Input: part model. Units: mm. Frame: model coordinates. A direction names the side the tool comes from. Give positions to 0.01 mm unless a question says otherwise; leave off trailing zeros. Loops run counter-clockwise (first coordinate to the right, second up) from the corner with the lowest first, then second, coordinate; pieces in that order, holes last. Notation, with made-up numbers: M 39,-7.75 L 59,-7.75 A20 cw 59,0.25 Z; hole C 44,63.25 d6. An arc over 180 degrees is marked long. Use CSV: the item, a comma, the result in double quotes. Start each with the question number.
Autodesk Inventor part; units mm, degrees
ref_plane "YZ Plane" through (0, 0, 0) normal (1, 0, 0) x (0, 1, 0)
ref_plane "XZ Plane" through (0, 0, 0) normal (0, 1, 0) x (-1, 0, 0)
ref_plane "XY Plane" through (0, 0, 0) normal (0, 0, 1) x (1, 0, 0)
sketch "Boceto1" plane through (0, 0, 0) normal (0, 0, 1) x (1, 0, 0)
  arc A0 (168.6959, -21.0168) -> (169.5218, -12.7418) centre (0, 0) ccw
  arc A1 (169.5218, -12.7418) -> (124.9741, 2.5458) centre (132.4533, -48.2091) ccw
  arc A2 (122.0053, -27.1977) -> (168.6959, -21.0168) centre (139.3691, 21.0776) ccw
  arc A3 (162.6596, 49.415) -> (160.0484, 57.3105) centre (0, 0) ccw
  arc A4 (160.0484, 57.3105) -> (113.134, 53.1573) centre (140.6105, 9.8324) ccw
  arc A5 (122.5196, 24.7777) -> (162.6596, 49.415) centre (118.7469, 75.9418) ccw
  arc A6 (128.4981, 111.3025) -> (122.9012, 117.4533) centre (0, 0) ccw
  arc A7 (122.9012, 117.4533) -> (81.7321, 94.5773) centre (124.4549, 66.1738) ccw
  arc A8 (101.8493, 72.4688) -> (128.4981, 111.3025) centre (77.5924, 117.6751) ccw
  arc A9 (72.1181, 153.9447) -> (64.5033, 157.2874) centre (0, 0) ccw
  arc A10 (64.5033, 157.2874) -> (36.1979, 119.6441) centre (86.7799, 111.0732) ccw
  arc A11 (63.5682, 107.6294) -> (72.1181, 153.9447) centre (23.0214, 139.0612) ccw
  arc A12 (3.2682, 169.9686) -> (-5.0479, 169.925) centre (0, 0) ccw
  arc A13 (-5.0479, 169.925) -> (-15.5952, 124.0233) centre (34.0998, 136.767) ccw
  arc A14 (14.2956, 124.1798) -> (3.2682, 169.9686) centre (-35.5302, 136.4024) ccw
  arc A15 (-66.1468, 156.6033) -> (-73.7262, 153.1811) centre (0, 0) ccw
  arc A16 (-73.7262, 153.1811) -> (-64.6918, 106.9578) centre (-24.4764, 138.8125) ccw
  arc A17 (-37.4488, 119.2585) -> (-66.1468, 156.6033) centre (-87.9383, 110.1584) ccw
  arc A18 (-124.1244, 116.1599) -> (-129.6566, 109.9508) centre (0, 0) ccw
  arc A19 (-129.6566, 109.9508) -> (-102.6026, 71.3983) centre (-78.8204, 116.8561) ccw
  arc A20 (-82.718, 93.7163) -> (-124.1244, 116.1599) centre (-125.141, 64.867) ccw
  arc A21 (-160.6398, 55.6314) -> (-163.1682, 47.7089) centre (0, 0) ccw
  arc A22 (-163.1682, 47.7089) -> (-122.7724, 23.4934) centre (-119.5357, 74.6942) ccw
  arc A23 (-113.6845, 51.9696) -> (-160.6398, 55.6314) centre (-140.7058, 8.3595) ccw
  arc A24 (-169.3791, -14.5163) -> (-168.4665, -22.7822) centre (0, 0) ccw
  arc A25 (-168.4665, -22.7822) -> (-121.7138, -28.4738) centre (-139.5821, 19.617) ccw
  arc A26 (-124.9939, 1.237) -> (-169.3791, -14.5163) centre (-131.9412, -49.5935) ccw
  arc A27 (-148.8312, -82.154) -> (-144.6355, -89.3341) centre (0, 0) ccw
  arc A28 (-144.6355, -89.3341) -> (-99.6097, -75.5175) centre (-135.4936, -38.8522) ccw
  arc A29 (-114.6907, -49.7095) -> (-148.8312, -82.154) centre (-100.3628, -98.9712) ccw
  arc A30 (-102.549, -135.5865) -> (-95.7956, -140.4393) centre (0, 0) ccw
  arc A31 (-95.7956, -140.4393) -> (-60.2823, -109.5036) centre (-107.9769, -90.6034) ccw
  arc A32 (-84.5565, -92.0608) -> (-102.549, -135.5865) centre (-51.4308, -131.2359) ccw
  arc A33 (-38.5352, -165.5749) -> (-30.3919, -167.2613) centre (0, 0) ccw
  arc A34 (-30.3919, -167.2613) -> (-10.5315, -124.5556) centre (-61.7901, -126.6885) ccw
  arc A35 (-39.8017, -118.494) -> (-38.5352, -165.5749) centre (6.3941, -140.8088) ccw
  arc A36 (32.1417, -166.9339) -> (40.267, -165.1623) centre (0, 0) ccw
  arc A37 (40.267, -165.1623) -> (41.0403, -118.0707) centre (-4.9192, -140.868) ccw
  arc A38 (11.8352, -124.4385) -> (32.1417, -166.9339) centre (63.1134, -126.0345) ccw
  arc A39 (97.261, -139.4285) -> (103.9632, -134.5052) centre (0, 0) ccw
  arc A40 (103.9632, -134.5052) -> (85.5159, -91.1703) centre (52.8023, -130.6902) ccw
  arc A41 (61.4257, -108.8664) -> (97.261, -139.4285) centre (108.9198, -89.4677) ccw
  arc A42 (145.563, -87.8146) -> (149.6833, -80.5909) centre (0, 0) ccw
  arc A43 (149.6833, -80.5909) -> (115.205, -48.5058) centre (101.3937, -97.9148) ccw
  arc A44 (100.3951, -74.4703) -> (145.563, -87.8146) centre (135.893, -37.4312) ccw
  arc A45 (113.134, 53.1573) -> (101.8493, 72.4688) centre (0, 0) ccw
  arc A46 (124.9741, 2.5458) -> (122.5196, 24.7777) centre (0, 0) ccw
  arc A47 (115.205, -48.5058) -> (122.0053, -27.1977) centre (0, 0) ccw
  arc A48 (85.5159, -91.1703) -> (100.3951, -74.4703) centre (0, 0) ccw
  arc A49 (41.0403, -118.0707) -> (61.4257, -108.8664) centre (0, 0) ccw
  arc A50 (-10.5315, -124.5556) -> (11.8352, -124.4385) centre (0, 0) ccw
  arc A51 (-60.2823, -109.5036) -> (-39.8017, -118.494) centre (0, 0) ccw
  arc A52 (-99.6097, -75.5175) -> (-84.5565, -92.0608) centre (0, 0) ccw
  arc A53 (-121.7138, -28.4738) -> (-114.6907, -49.7095) centre (0, 0) ccw
  arc A54 (-122.7724, 23.4934) -> (-124.9939, 1.237) centre (0, 0) ccw
  arc A55 (-102.6026, 71.3983) -> (-113.6845, 51.9696) centre (0, 0) ccw
  arc A56 (-64.6918, 106.9578) -> (-82.718, 93.7163) centre (0, 0) ccw
  arc A57 (-15.5952, 124.0233) -> (-37.4488, 119.2585) centre (0, 0) ccw
  arc A58 (81.7321, 94.5773) -> (63.5682, 107.6294) centre (0, 0) ccw
  arc A59 (36.1979, 119.6441) -> (14.2956, 124.1798) centre (0, 0) ccw
  dimension "d8" = 360
extrude "Extrusión1" add sketch "Boceto1" along normal blind 30
properties part number "15P_Recto"
Item 1: Section B-B (y = -65). Output: boundary loops of the cut face in (x, z), then the cut area to 3 significant figures.
Item 2: Material intervals for line 1 (Y direction, x = -122.5, z = 3.75); line 2 (Y direction, x = -135, z = 23); line 3 (X direction, y = 135, z = 15.25), sorted ascending.
Item 3: Set-up query: faces 5 (the cylindrical face through (-120.62, 87.11, 14.79)), 6 (the cylindrical face through (72.82, 101.6, 14.79)). Return all of +Z, -Z, +X, -X, +Y, -Y with unobstructed straight access to the full face (end or side cutting, diameter ignored); none if empty.
Item 4: First-contact query: pin 1 Ø2 at (y, z) = (21.5, 5.5) entering from -X; pin 2 Ø8 at (y, z) = (-87, 8) entering from -X; pin 3 Ø3 at (x, z) = (13, 26) entering from +Y. Flat tips, straight axial feed; report the tip coordinate or a pass-through.
Item 5: Mould query, pull axis X, two halves, no side actions, for faces 1 (the cylindrical face through (-47.47, 141.69, 14.79)), 2 (the cylindrical face through (169.165, -16.826, 14.79)), 3 (the cylindrical face through (16.97, -148.46, 14.79)), 4 (the flat face through (-2, 4, 0)). Classes: +X half, -X half, draft (parallel to the pull), parting line (faces both ways), or undercut.
Item 6: Section A-A (y = 67.5). Output: boundary loops of the cut face in (x, z), then the cut area to 3 significant figures.
Recorded:
1,outline,"M -138.81,0 L 140.75,0 L 140.75,30 L -138.81,30 Z"
1,area,"8,390 mm²"
2,line 1,"-88.48 to -52.69, -28.76 to 56.32, 89.95 to 116.1"
2,line 2,"-90.15 to -61.13, -31.48 to 1.62, 25.78 to 59.34"
2,line 3,"-75.64 to -43.05, -17.17 to 15.75, 41.4 to 74.16"
3,face 5,"+Z, -Z, -X"
3,face 6,"+Z, -Z"
4,pin 1,"x = -123.31"
4,pin 2,"x = -148.36"
4,pin 3,"y = 156.9"
5,face 1,"undercut"
5,face 2,"+X half"
5,face 3,"undercut"
5,face 4,"draft"
6,outline,"M -105.21,0 L 105.21,0 L 105.21,30 L -105.21,30 Z"
6,area,"6,310 mm²"
